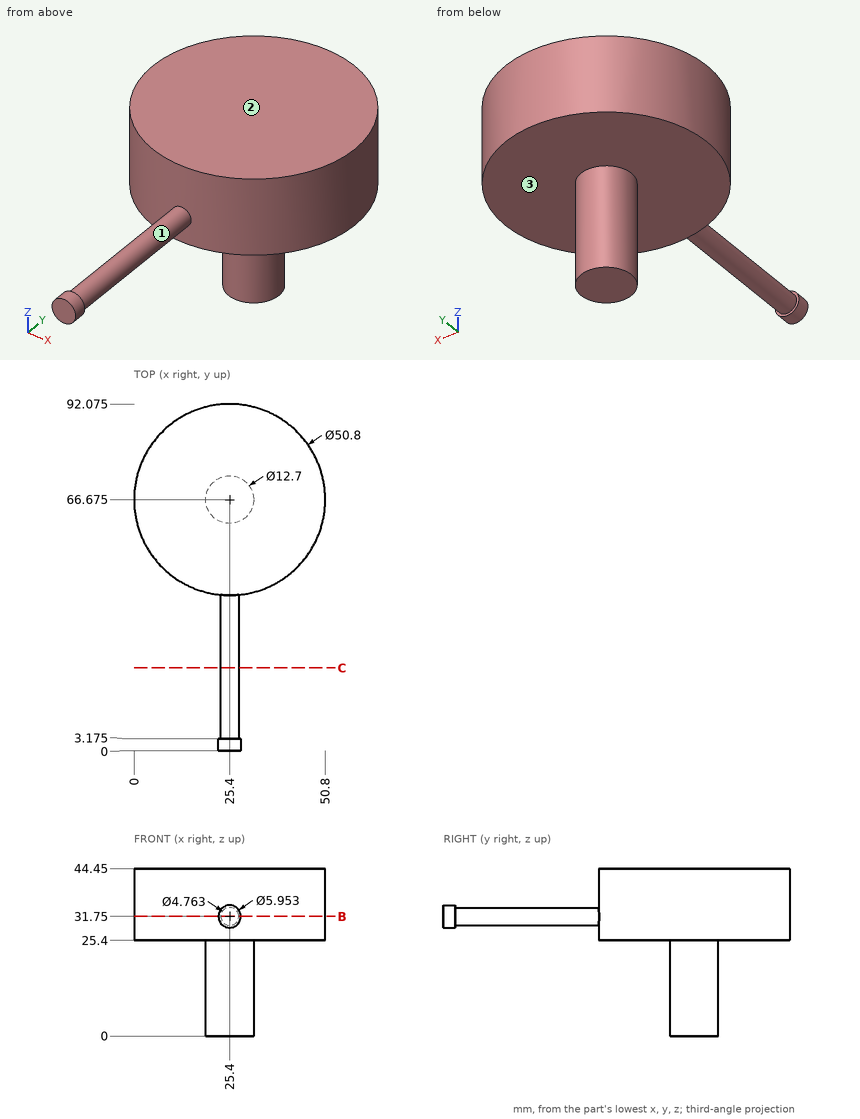
Source: three-view drawing plus pictorial views. Frame: mm from the lowest corner of the part. A direction names the side the tool comes from. Give positions to 0.01 mm unless a question says otherwise; leave off trailing zeros. Order: outer loops, then holes, each group sorted by start corner. A loop starts at its lowest first (then second) coordinate and runs counter-clockwise, first axis right, second up. Notation, with made-up numbers: M 75,50.5 L 93,50.5 A10 cw 93,54.5 Z; hole C 64.25,57 d5. An arc over 180 degrees is marked long. Return JSON: item names as keys, results as strings.
Item 1: Access query for the marked faces 1, 2 and 3. Directions: +Z, -Z, +X, -X, +Y, -Y. A direction counts if a zero-diameter tool reaches every point of the face in a straight line with its end or side. Return the directions, or none.
Solutions:
{"face 1": "none", "face 2": "+Z, +X, -X, +Y, -Y", "face 3": "-Z"}
Item 2: First-contact query: P1, Ø8, axis at y = 69.5, z = 17, coming from the -X side; P2, Ø8, axis at x = 28.5, z = 16, coming from the -Y side (1 decimal); P3, Ø8, axis at y = 79.5, z = 22.5, coming from the +X side. Flat tips, straight axial feed; report the tip coordinate or a pass-through.
Solutions:
{"P1": "x = 19.05", "P2": "y = 60.3", "P3": "x = 48.72"}
Item 3: Cut plane B-B (z = 31.75). Return loops of the section in (x, y) (1 decimal).
Solutions:
{"outline": "M 22.4,0 L 28.4,0 L 28.4,3.2 L 27.8,3.2 L 27.8,41.4 A25.4 ccw long 23,41.4 L 23,3.2 L 22.4,3.2 Z"}
Item 4: Cut plane C-C (y = 22). Return loops of the section in (x, z).
Solutions:
{"outline": "C 25.4,31.75 d4.76"}
Item 5: Ray query, probe 1 along Z at (x, y) = (45.5, 71); probe 2 along Y at (x, z) = (20.5, 12) (1 decimal); probe 3 along X at (y, z) = (68, 40.5) (1 decimal). Return the intervals inside material, ascending.
Solutions:
{"probe 1": "25.4 to 44.45", "probe 2": "62.6 to 70.7", "probe 3": "0 to 50.8"}
